The drawing under review shows one solid part. Ordinate dimensions are in mm from its lowest x, y, z. A direction names the side the tool comes from. Round coordinates to 2 decimals unless told otherwise and drop trailing zeros. Loops run counter-clockwise (first coordinate to the right, second up) from the corner with the lowest first, then second, coordinate; pieces in that order, holes last. Notation, with made-up numbers: (-39, 24) - (-18, 24) arc R11 ccw to (-18, 38) - close; hole circle Ø10 at (69.5, 85). An arc over 180 degrees is marked (long way). Answer as CSV lines item,"result".
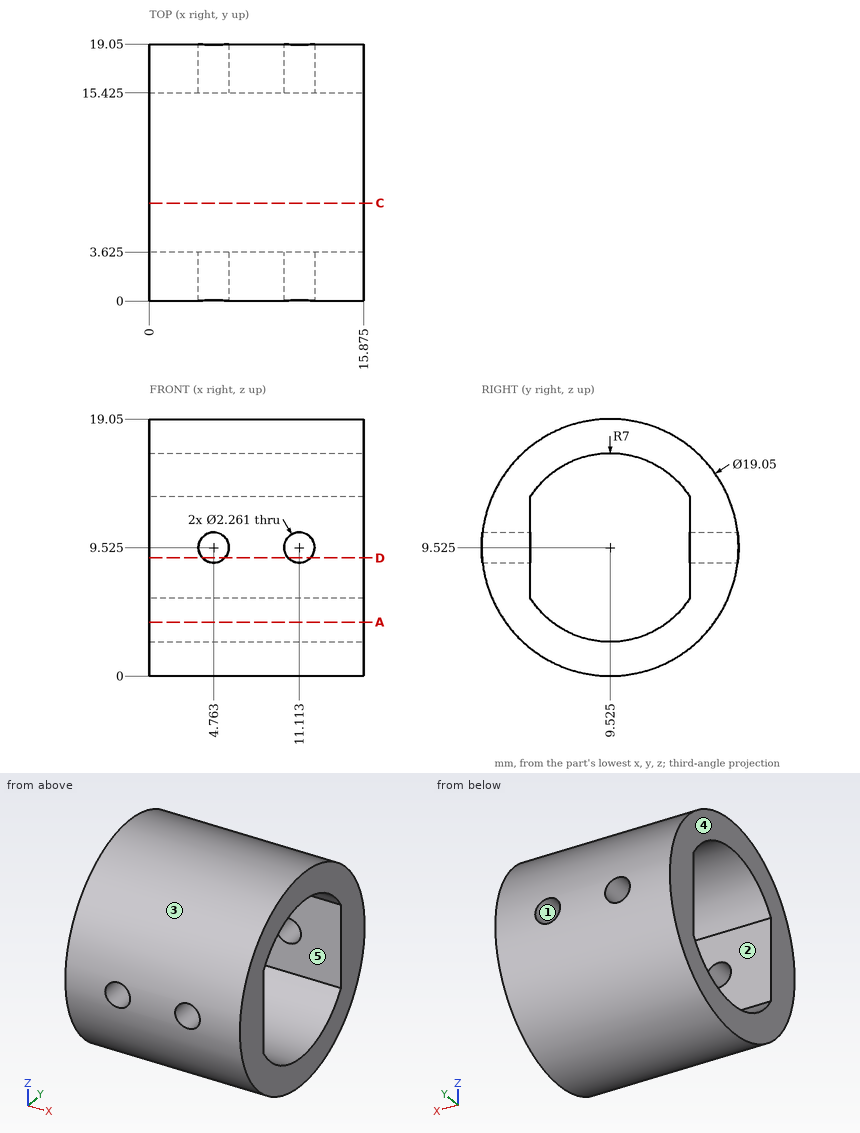
1. Clearance check with flat-ended pins moving along their axes: pin 1 (1 mm diameter, centred on x = 3, y = 5.5, fed in from -Z); pin 2 (1.8 mm diameter, centred on x = 4.76, z = 9.53, fed in from -Y); pin 3 (6 mm diameter, centred on x = 11, y = 14.5, fed in from -Z). State where each tip first meets the part, or that it passes through.
Numbers:
pin 1,"stops at z = 0.68"
pin 2,"passes through"
pin 3,"stops at z = 0.21"
2. Tool access review of the marked faces 1 and 2: name each direction out of +Z, -Z, +X, -X, +Y, -Y from which nothing blocks a thin tool from reaching the whole face with its end or side.
Numbers:
face 1,"+Y, -Y"
face 2,"+X, -X"
3. Take a section at C-C (y = 7.25). State the section outline as (x, z) points (1 decimal).
Numbers:
outline,"(0, 0.3) - (15.9, 0.3) - (15.9, 2.9) - (0, 2.9) - close; (0, 16.1) - (15.9, 16.1) - (15.9, 18.8) - (0, 18.8) - close"
4. Draft analysis for pull direction Y (two halves, no side actions). For the marked faces 3, 4 and 5, state which applies: +Y half, -Y half, draft (parallel to the pull), parting line (faces both ways), or undercut.
Numbers:
face 3,"parting line"
face 4,"draft"
face 5,"undercut"
5. Wall thickness on probe 1 along Y at (x, z) = (12, 8.75) (1 decimal); probe 2 along Z at (x, y) = (1.25, 8.25) (1 decimal); probe 3 along Y at (x, z) = (11.5, 11) (1 decimal): over which ranges is each line inside the solid? List them lowest first.
Numbers:
probe 1,"y = 0 to 3.6, 15.4 to 19"
probe 2,"z = 0.1 to 2.6, 16.4 to 19"
probe 3,"y = 0.1 to 3.6, 15.4 to 18.9"
6. Take a section at D-D (z = 8.75). State the section outline as (x, y) points (1 decimal).
Numbers:
outline,"(0, 0) - (3.9, 0) - (3.9, 3.6) - (0, 3.6) - close; (0, 15.4) - (3.9, 15.4) - (3.9, 19) - (0, 19) - close; (5.6, 0) - (10.3, 0) - (10.3, 3.6) - (5.6, 3.6) - close; (5.6, 15.4) - (10.3, 15.4) - (10.3, 19) - (5.6, 19) - close; (11.9, 0) - (15.9, 0) - (15.9, 3.6) - (11.9, 3.6) - close; (11.9, 15.4) - (15.9, 15.4) - (15.9, 19) - (11.9, 19) - close"
7. Take a section at A-A (z = 4). State the section outline as (x, y) points (1 decimal).
Numbers:
outline,"(0, 1.8) - (15.9, 1.8) - (15.9, 5.2) - (0, 5.2) - close; (0, 13.8) - (15.9, 13.8) - (15.9, 17.3) - (0, 17.3) - close"
